Part model, mm, in its own coordinate system. Face numbers are marked on the shaded views. A direction names the side the tool comes from. Round coordinates to 2 decimals unless told otherwise and drop trailing zeros. Loops run counter-clockwise (first coordinate to the right, second up) from the corner with the lowest first, then second, coordinate; pieces in that order, holes last. Notation, with made-up numbers: (67.5, -7) -> (82.5, -7) arc R18 ccw to (82.5, 12) -> close; hole circle Ø8 at (80.25, -19.5). An arc over 180 degrees is marked (long way). Use a Markdown table: item, result. Add a question column.
Item 1: Cut at B-B, the plane z = 17.75. List the corners of the cut face in (x, y).
Item 2: Cut at D-D, the plane z = 9. List the corners of the cut face in (x, y), plus the area to 3 significant figures.
Item 3: Which spindle directions (+Z, -Z, +X, -X, +Y, -Y) get a long thin tool onto all of the face, cutting with end or side? Do the marked faces 1, 2, 3 and 4. Say none if no direction does.
Item 4: Two-plate mould, pull along X, no slides. Class the marked faces 5, 6, 7 and 8: pulls with the +X half, pulls with the -X half, needs draft (parallel to the pull), parting line crosses it, or undercut.
Item 5: Probe line 1 (X direction, y = 10, z = 13.25); line 2 (Z direction, x = 32.5, y = 3.5); line 3 (X direction, y = -5.75, z = 15). List the from-to ranges inside material, lowest first. Write a range as [from, to].
Item 6: Flat gauge pins, fed straight in: pin 1 (4 mm diameter, centred on x = 11.5, z = 14.5, fed in from +Y); pin 2 (6.5 mm diameter, centred on x = 30, y = 2, fed in from +Z); pin 3 (2 mm diameter, centred on y = 7, z = 9.5, fed in from -X). Where does each tip first touch, or does it go through?
Item 7: Cut at A-A, the plane y = 0. List the corners of the cut face in (x, z), plus the area to 3 significant figures.
Item 8: Cut at C-C, the plane x = 11. List the corners of the cut face in (y, z).
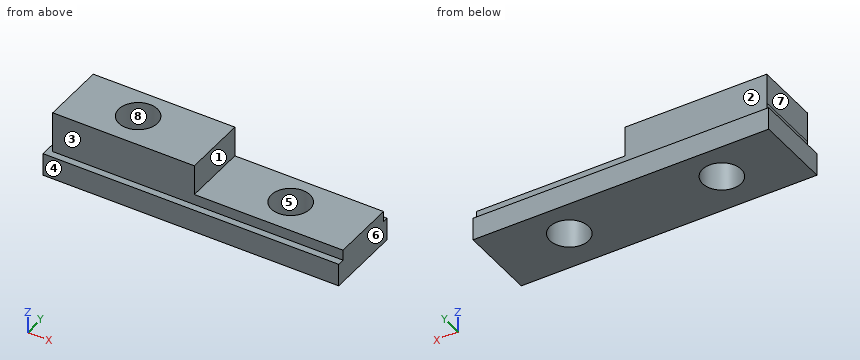
```python
from build123d import *

# Parameters (mm, degrees)
F0_W     = 98.998546
F0_H     = 25.809678
F1_DEPTH = 7.62
F2_W     = 97.194314
F2_H     = 21.661694
F3_DEPTH = 3.556
F4_W     = 47.418509
F4_H     = 21.661694
F5_DEPTH = 10.16
F6_R     = 6.469009
F6_R_2   = 6.469136
F7_DEPTH = 21.844


with BuildPart() as f1:
    # F0 (on Top) → F1 (new body)
    with BuildSketch(Plane.XY):
        with Locations((0.276532, -0.921774)):
            Rectangle(F0_W, F0_H)
    extrude(amount=F1_DEPTH)

    # F2 (on face) → F3 (join)
    with BuildSketch(Plane.XY.offset(7.62)):
        with Locations((1.178648, -0.691053)):
            Rectangle(F2_W, F2_H)
    extrude(amount=F3_DEPTH)

    # F4 (on face) → F5 (join)
    with BuildSketch(Plane.XY.offset(11.176)):
        with Locations((-23.709255, -0.691053)):
            Rectangle(F4_W, F4_H)
    extrude(amount=F5_DEPTH)

    # F6 (on face) → F7 (cut)
    with BuildSketch(Plane.XY.offset(21.336)):
        with Locations((-26.033347, 0)):
            Circle(F6_R)
        with Locations((25.032943, 0)):
            Circle(F6_R_2)
    extrude(amount=-F7_DEPTH, mode=Mode.SUBTRACT)


solid = f1.part
```
A:
| question | item | result |
|---|---|---|
| 1 | outline | (-47.42, -11.52) -> (0, -11.52) -> (0, 10.14) -> (-47.42, 10.14) -> close; hole circle Ø12.94 at (-26.03, 0) |
| 2 | outline | (-47.42, -11.52) -> (49.78, -11.52) -> (49.78, 10.14) -> (-47.42, 10.14) -> close; hole circle Ø12.94 at (-26.03, 0); hole circle Ø12.94 at (25.03, 0) |
| 2 | area | 1,840 mm^2 |
| 3 | face 1 | +Z, +X, +Y, -Y |
| 3 | face 2 | +Z, +X, -X, +Y |
| 3 | face 3 | +Z, +X, -X, -Y |
| 3 | face 4 | +Z, -Z, +X, -X, -Y |
| 4 | face 5 | undercut |
| 4 | face 6 | pulls with the +X half |
| 4 | face 7 | pulls with the -X half |
| 4 | face 8 | undercut |
| 5 | line 1 | x = [-47.42, 0] |
| 5 | line 2 | z = [0, 11.18] |
| 5 | line 3 | x = [-47.42, -29], [-23.07, 0] |
| 6 | pin 1 | passes through |
| 6 | pin 2 | stops at z = 11.18 |
| 6 | pin 3 | stops at x = -47.42 |
| 7 | outline | (-49.22, 0) -> (-32.5, 0) -> (-32.5, 21.34) -> (-47.42, 21.34) -> (-47.42, 7.62) -> (-49.22, 7.62) -> close; (-19.56, 0) -> (18.56, 0) -> (18.56, 11.18) -> (0, 11.18) -> (0, 21.34) -> (-19.56, 21.34) -> close; (31.5, 0) -> (49.78, 0) -> (49.78, 11.18) -> (31.5, 11.18) -> close |
| 7 | area | 1,160 mm^2 |
| 8 | outline | (-13.83, 0) -> (11.98, 0) -> (11.98, 7.62) -> (10.14, 7.62) -> (10.14, 11.18) -> (-11.52, 11.18) -> (-11.52, 7.62) -> (-13.83, 7.62) -> close |
